Geometry check sheet. Reference: the model listing, model coordinates, mm. Face numbers are marked on the shaded views. A direction names the side the tool comes from. Coordinates: 2 decimals unless noted, no trailing zeros. Write each loop counter-clockwise with the first axis right and the second up, starting at its lowest first coordinate (ties: lowest second). Pieces come first, ordered by that corner, then holes. Notation, with made-up numbers: M 4,-20 L 35,-20 A26 ccw 35,8 Z; hole C 74,3 d4. An arc over 180 degrees is marked long. Answer as a JSON object with one key per item and string values. Group by question number.
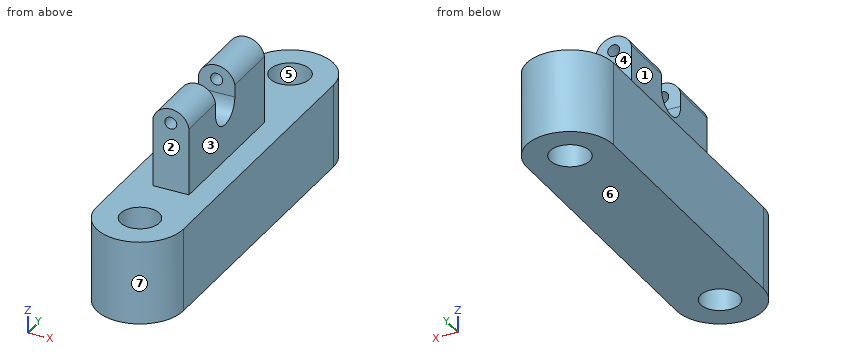
```python
from build123d import *

# Parameters (mm, degrees)
F0_R     = 2.9421946195
F0_R_2   = 3.0131155992
F1_DEPTH = 12.7
F2_W     = 5.4983180016
F2_H     = 22.1828678623
F3_DEPTH = 25.4
F5_DEPTH = 25.4
F7_DEPTH = 127
F8_R     = 0.907588381
F9_DEPTH = 127


with BuildPart() as f1:
    # F0 (on Top) → F1 (new body)
    with BuildSketch(Plane.XY):
        with BuildLine():
            Line((0, 44.08133775), (0, 0))
            ThreePointArc((0, 0), (6.5885009244, -6.5885009244), (13.1770018488, 0))
            Line((13.1770018488, 0), (13.1770018488, 44.08133775))
            ThreePointArc((13.1770018488, 44.08133775), (6.5885009244, 50.6698386744), (0, 44.08133775))
        make_face()
        with Locations((6.5885009244, 0)):
            Circle(F0_R, mode=Mode.SUBTRACT)
        with Locations((6.5885009244, 44.08133775)):
            Circle(F0_R_2, mode=Mode.SUBTRACT)
    extrude(amount=F1_DEPTH)

    # F2 (on Top) → F3 (join)
    with BuildSketch(Plane.XY):
        with Locations((6.8254983053, 19.7181045078)):
            Rectangle(F2_W, F2_H)
    extrude(amount=F3_DEPTH)

    # F4 (on face) → F5 (cut)
    with BuildSketch(Plane.YZ.offset(9.5746573061)):
        with BuildLine():
            Line((22.0856051892, 25.4), (16.4166372269, 25.4))
            Line((16.4166372269, 25.4), (16.4166372269, 21.0717450827))
            ThreePointArc((16.4166372269, 21.0717450827), (19.2511212081, 18.2372611016), (22.0856051892, 21.0717450827))
            Line((22.0856051892, 21.0717450827), (22.0856051892, 25.4))
        make_face()
    extrude(amount=-F5_DEPTH, mode=Mode.SUBTRACT)

    # F6 (on face) → F7 (cut)
    with BuildSketch(Plane.XZ.offset(-8.6266705766)):
        with BuildLine():
            ThreePointArc((4.0763393044, 23.1695235286), (6.9185308411, 25.3015410804), (9.5746573061, 22.9417648677))
            Line((9.5746573061, 22.9417648677), (9.5746573061, 25.4))
            Line((9.5746573061, 25.4), (8.0125611275, 25.4))
            Line((8.0125611275, 25.4), (5.4706284103, 25.4))
            Line((5.4706284103, 25.4), (4.0763393044, 25.4))
            Line((4.0763393044, 25.4), (4.0763393044, 23.5414523631))
            Line((4.0763393044, 23.5414523631), (4.0763393044, 23.1695235286))
        make_face()
    extrude(amount=-F7_DEPTH, mode=Mode.SUBTRACT)

    # F8 (on face) → F9 (cut)
    with BuildSketch(Plane.XZ.offset(-8.6266705766)):
        with Locations((6.8111866713, 23.1206584722)):
            Circle(F8_R)
    extrude(amount=-F9_DEPTH, mode=Mode.SUBTRACT)


solid = f1.part
```
1) Go/stop test with flat-tipped pins: pin 1 Ø2.5 at (x, z) = (5.5, 18) entering from +Y; pin 2 Ø3.5 at (x, z) = (6, 23) entering from -Y; pin 3 Ø1 at (y, z) = (18, 19) entering from +X. Record where each tip stops, or that it passes through.
2) Section check A-A (y = 46.5). Record the cut outline in (x, z).
3) Draft check along Y on the marked faces 4, 5, 6 and 7. Enter one of: +Y half, -Y half, draft (parallel to the pull), parting line (faces both ways), or undercut.
4) Material ranges on probe 1 along Z at (x, y) = (2, 45); probe 2 along Y at (x, z) = (8.75, 10); probe 3 along Y at (x, z) = (4.25, 20.25), recorded low to high. Write a range as [from, to].
5) Set-up check for the marked faces 1, 2 and 3: record each of +Z, -Z, +X, -X, +Y, -Y from which the full face is reachable in a straight line by a thin tool's end or side.
6) Section check D-D (x = 12). Record the cut outline in (y, z), then the cut area to 3 significant figures.
7) Section check B-B (x = 4.75). Record the cut outline in (y, z), then the cut area to 3 significant figures.
8) Section check C-C (y = 18). Record the cut outline in (x, z).
Entries:
{
 "1": {"pin 1": "y = 30.81", "pin 2": "y = 8.63", "pin 3": "x = 9.57"},
 "2": {"outline": "M 0.46,0 L 4.79,0 L 4.79,12.7 L 0.46,12.7 Z; M 8.39,0 L 12.72,0 L 12.72,12.7 L 8.39,12.7 Z"},
 "3": {"face 4": "+Y half", "face 5": "undercut", "face 6": "draft", "face 7": "-Y half"},
 "4": {"probe 1": "[0, 12.7]", "probe 2": "[-6.22, -2], [2, 41.98], [46.18, 50.31]", "probe 3": "[8.63, 16.54], [21.96, 30.81]"},
 "5": {"face 1": "+Z, -X, +Y, -Y", "face 2": "+Z, +X, -X, -Y", "face 3": "+Z, +X, +Y, -Y"},
 "6": {"outline": "M -3.76,0 L 47.84,0 L 47.84,12.7 L -3.76,12.7 Z", "area": "655 mm^2"},
 "7": {"outline": "M -6.33,0 L -2.3,0 L -2.3,12.7 L -6.33,12.7 Z; M 2.3,0 L 41.69,0 L 41.69,12.7 L 30.81,12.7 L 30.81,24.41 L 22.09,24.41 L 22.09,21.07 A2.83 cw 16.42,21.07 L 16.42,24.41 L 8.63,24.41 L 8.63,12.7 L 2.3,12.7 Z; M 46.47,0 L 50.41,0 L 50.41,12.7 L 46.47,12.7 Z", "area": "830 mm^2"},
 "8": {"outline": "M 0,0 L 13.18,0 L 13.18,12.7 L 9.57,12.7 L 9.57,18.53 L 4.08,18.53 L 4.08,12.7 L 0,12.7 Z"}
}
